Check sheet for the modelled part. Datum: model origin and axes. Units: mm. Face numbers are marked on the shaded views. A direction names the side the tool comes from. Round coordinates to 2 decimals unless told otherwise and drop trailing zeros. Loops run counter-clockwise (first coordinate to the right, second up) from the corner with the lowest first, then second, coordinate; pieces in that order, holes last. Notation, with made-up numbers: (58.25, 51) - (79.25, 51) arc R25 cw to (79.25, 77) - close; hole circle Ø9 at (60, 65.5). An arc over 180 degrees is marked (long way). Put each result on its own line as item: value.
```python
from build123d import *

# Parameters (mm, degrees)
SKETCH1_R           = 67.5
BOSS_EXTRUDE1_DEPTH = 15
SKETCH2_R           = 47.25
SKETCH2_R_2         = 25
CUT_EXTRUDE1_DEPTH  = 6
CUT_EXTRUDE2_DEPTH  = 10
SKETCH5_R           = 2.5
CUT_EXTRUDE3_DEPTH  = 10
SKETCH6_R           = 2
CUT_EXTRUDE4_DEPTH  = 15
SKETCH7_R           = 5
CUT_EXTRUDE5_DEPTH  = 5
SKETCH8_R           = 2
CUT_EXTRUDE6_DEPTH  = 10


with BuildPart() as part:
    # Sketch1 → Boss-Extrude1 (new body)
    with BuildSketch(Plane(origin=(0, 0, 0), x_dir=(1, 0, 0), z_dir=(0, 1, 0))):
        Circle(SKETCH1_R)
    extrude(amount=BOSS_EXTRUDE1_DEPTH)

    # Sketch2 → Cut-Extrude1 (cut)
    with BuildSketch(Plane(origin=(0, 15, 0), x_dir=(1, 0, 0), z_dir=(0, 1, 0))):
        Circle(SKETCH2_R)
        Circle(SKETCH2_R_2, mode=Mode.SUBTRACT)
    extrude(amount=-CUT_EXTRUDE1_DEPTH, mode=Mode.SUBTRACT)

    # Sketch3 → Cut-Extrude2 (cut)
    with BuildSketch(Plane(origin=(0, 15, 0), x_dir=(1, 0, 0), z_dir=(0, 1, 0))):
        with BuildLine():
            Line((-9, 8.960468738), (-9, -8.960468738))
            ThreePointArc((-9, -8.960468738), (12.7, 0), (-9, 8.960468738))
        make_face()
    extrude(amount=-CUT_EXTRUDE2_DEPTH, mode=Mode.SUBTRACT)

    # Sketch5 → Cut-Extrude3 (cut)
    with BuildSketch(Plane(origin=(0, 5, 0), x_dir=(1, 0, 0), z_dir=(0, 1, 0))):
        Circle(SKETCH5_R)
    extrude(amount=-CUT_EXTRUDE3_DEPTH, mode=Mode.SUBTRACT)

    # Sketch6 → Cut-Extrude4 (cut)
    with BuildSketch(Plane(origin=(0, 15, 0), x_dir=(1, 0, 0), z_dir=(0, 1, 0))):
        with Locations((0, 57.5)):
            Circle(SKETCH6_R)
        with Locations((49.796460718, 28.75)):
            Circle(SKETCH6_R)
        with Locations((49.796460718, -28.75)):
            Circle(SKETCH6_R)
        with Locations((0, -57.5)):
            Circle(SKETCH6_R)
        with Locations((-49.796460718, -28.75)):
            Circle(SKETCH6_R)
        with Locations((-49.796460718, 28.75)):
            Circle(SKETCH6_R)
    extrude(amount=-CUT_EXTRUDE4_DEPTH, mode=Mode.SUBTRACT)

    # Sketch7 → Cut-Extrude5 (cut)
    with BuildSketch(Plane(origin=(0, 15, 0), x_dir=(1, 0, 0), z_dir=(0, 1, 0))):
        with Locations((0, 57.5)):
            Circle(SKETCH7_R)
        with Locations((49.796460718, 28.75)):
            Circle(SKETCH7_R)
        with Locations((49.796460718, -28.75)):
            Circle(SKETCH7_R)
        with Locations((0, -57.5)):
            Circle(SKETCH7_R)
        with Locations((-49.796460718, -28.75)):
            Circle(SKETCH7_R)
        with Locations((-49.796460718, 28.75)):
            Circle(SKETCH7_R)
    extrude(amount=-CUT_EXTRUDE5_DEPTH, mode=Mode.SUBTRACT)

    # Sketch8 → Cut-Extrude6 (cut)
    with BuildSketch(Plane.XZ):
        with Locations((-25, 45)):
            Circle(SKETCH8_R)
        with Locations((-45, 45)):
            Circle(SKETCH8_R)
        with Locations((25, 45)):
            Circle(SKETCH8_R)
        with Locations((45, 45)):
            Circle(SKETCH8_R)
        with Locations((45, -45)):
            Circle(SKETCH8_R)
        with Locations((25, -45)):
            Circle(SKETCH8_R)
        with Locations((-25, -45)):
            Circle(SKETCH8_R)
        with Locations((-45, -45)):
            Circle(SKETCH8_R)
    extrude(amount=-CUT_EXTRUDE6_DEPTH, mode=Mode.SUBTRACT)


solid = part.part
```
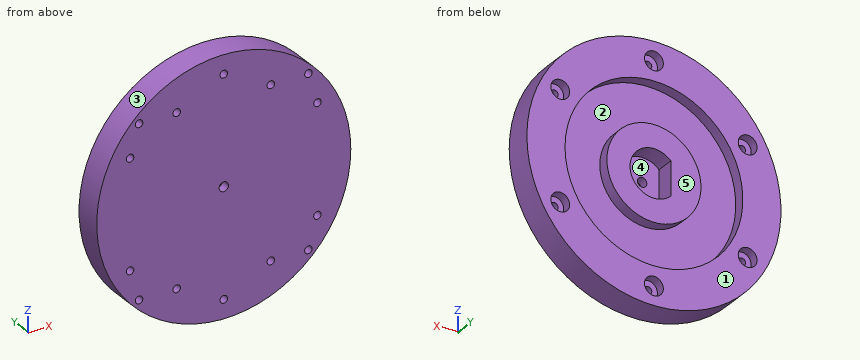
Item 1: Section check B-B on y = 7.25. Count the separate pieces of the cut face and the enclosed holes in it, then the cut area to 3 significant figures.
Filled sheet:
separate pieces: 1
enclosed holes: 15
area: 13,700 mm²
Item 2: Section check A-A on z = 0. Enter the section's corners in (x, y), then the cut area to 3 significant figures.
Filled sheet:
outline: (-67.5, 0) - (-2.5, 0) - (-2.5, 5) - (-9, 5) - (-9, 15) - (-25, 15) - (-25, 9) - (-47.25, 9) - (-47.25, 15) - (-67.5, 15) - close; (2.5, 0) - (67.5, 0) - (67.5, 15) - (47.25, 15) - (47.25, 9) - (25, 9) - (25, 15) - (12.7, 15) - (12.7, 5) - (2.5, 5) - close
area: 1,520 mm²
Item 3: Tool access check on the marked faces 1 and 2. Record the directions out of +Z, -Z, +X, -X, +Y, -Y that give a thin tool (end or side, any length) a straight path to the whole face; none if there is none.
Filled sheet:
face 1: +Z, -Z, +X, -X, +Y
face 2: +Y
Item 4: Release check for a two-part mould opening along Z. For the marked faces 3, 4 and 5 record: +Z half, -Z half, draft (parallel to the pull), parting line (faces both ways), or undercut.
Filled sheet:
face 3: parting line
face 4: undercut
face 5: draft
Item 5: Section check C-C on x = -20.5. Enter the section's corners in (y, z).
Filled sheet:
outline: (0, -64.31) - (15, -64.31) - (15, -42.57) - (9, -42.57) - (9, -14.31) - (15, -14.31) - (15, 14.31) - (9, 14.31) - (9, 42.57) - (15, 42.57) - (15, 64.31) - (0, 64.31) - close
Item 6: Thickness scan on line 1 (Z direction, x = -45, y = 2); line 2 (Z direction, x = 0, y = 5.25); line 3 (Z direction, x = -25, y = 7.5). Record the ranges inside material, lowest first. Write a range as from..to.
Filled sheet:
line 1: -50.31..-47, -43..43, 47..50.31
line 2: -67.5..-59.5, -55.5..-12.7, 12.7..55.5, 59.5..67.5
line 3: -62.7..-47, -43..43, 47..62.7
Item 7: Section check D-D on z = -39. Enter the section's corners in (x, y).
Filled sheet:
outline: (-55.09, 0) - (55.09, 0) - (55.09, 15) - (26.68, 15) - (26.68, 9) - (-26.68, 9) - (-26.68, 15) - (-55.09, 15) - close
Item 8: Go/stop test with flat-tipped pins: pin 1 (8 mm diameter, centred on x = -0.5, z = 14, fed in from -Y); pin 2 (4 mm diameter, centred on x = -25.5, y = 4, fed in from -Z); pin 3 (5 mm diameter, centred on x = -41.5, y = 13, fed in from -Z); pin 4 (3 mm diameter, centred on y = 12.5, z = 6, fed in from -X). Record where each tip stops, or that it passes through.
Filled sheet:
pin 1: y = 0
pin 2: z = -63.28
pin 3: z = -55.09
pin 4: x = -67.35
